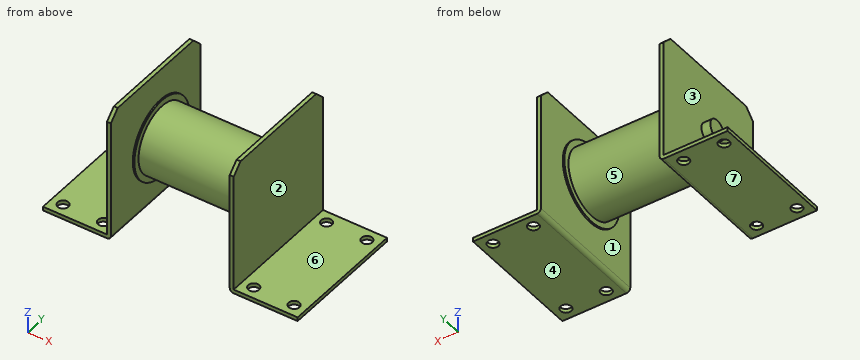
```python
from build123d import *

# Parameters (mm, degrees)
F0_R          = 20
F1_DEPTH      = 27.8
F1_DEPTH_BACK = 27.8
F2_R          = 7
F3_DEPTH      = 28.8
F3_DEPTH_BACK = 28.8
F4_R          = 20
F4_R_2        = 17
F5_DEPTH      = 27
F5_DEPTH_BACK = 27
F6_R          = 5
F7_DEPTH      = 32.2
F7_DEPTH_BACK = 36.7
F9_DEPTH      = 32.5
F9_DEPTH_BACK = 32.5
F10_SIZE      = 5
F11_R         = 2
F13_D         = 5.5


with BuildPart() as f1:
    # F0 (on Right) → F1 (new body, two sides)
    with BuildSketch(Plane.YZ) as f1_sk:
        Circle(F0_R)
    extrude(amount=F1_DEPTH)
    extrude(f1_sk.sketch, amount=-F1_DEPTH_BACK)

    # F2 (on Right) → F3 (join, two sides)
    with BuildSketch(Plane.YZ) as f3_sk:
        Circle(F2_R)
    extrude(amount=F3_DEPTH)
    extrude(f3_sk.sketch, amount=-F3_DEPTH_BACK)

    # F4 (on Right) → F5 (cut, two sides)
    with BuildSketch(Plane.YZ) as f5_sk:
        Circle(F4_R)
        Circle(F4_R_2, mode=Mode.SUBTRACT)
    extrude(amount=-F5_DEPTH, mode=Mode.SUBTRACT)
    extrude(f5_sk.sketch, amount=F5_DEPTH_BACK, mode=Mode.SUBTRACT)

    # F6 (on Right) → F7 (join, two sides)
    with BuildSketch(Plane.YZ) as f7_sk:
        Circle(F6_R)
    extrude(amount=F7_DEPTH)
    extrude(f7_sk.sketch, amount=-F7_DEPTH_BACK)

    # F8 (on Front) → F9 (join, two sides)
    with BuildSketch(Plane.XZ) as f9_sk:
        Polygon((32.2, 32.5), (30.2, 32.5), (30.2, -34.5), (64.7, -34.5), (64.7, -32.5), (32.2, -32.5), align=None)
        Polygon((-30.2, -34.5), (-30.2, 32.5), (-32.2, 32.5), (-32.2, -32.5), (-64.7, -32.5), (-64.7, -34.5), align=None)
    extrude(amount=F9_DEPTH)
    extrude(f9_sk.sketch, amount=-F9_DEPTH_BACK)

    # F10
    f10_edges = [f1.edges().sort_by_distance(p)[0] for p in [
        (31.2, -32.5, 32.5),
        (31.2, 32.5, 32.5),
        (-31.2, -32.5, 32.5),
        (-31.2, 32.5, 32.5),
    ]]
    chamfer(f10_edges, length=F10_SIZE)

    # F11
    f11_edges = [f1.edges().sort_by_distance(p)[0] for p in [
        (30.2, 0, -34.5),
        (-30.2, 0, -34.5),
    ]]
    fillet(f11_edges, radius=F11_R)

    # F13 (through all)
    with Locations(Plane.XY.offset(-32.5)):
        with Locations((38.2, 26.5), (38.2, -26.5), (58.7, -26.5), (-38.2, -26.5), (-58.7, -26.5), (-58.7, 26.5), (-38.2, 26.5), (58.7, 26.5)):
            Hole(F13_D / 2)


solid = f1.part
```
CAD build for the part. Positions are in the model's coordinates, mm. Face numbers are marked on the shaded views. A direction names the side the tool comes from. Round coordinates to 2 decimals unless told otherwise and drop trailing zeros. Write each loop counter-clockwise with the first axis right and the second up, starting at its lowest first coordinate (ties: lowest second). Pieces come first, ordered by that corner, then holes. Notation, with made-up numbers: (43.25, 28) - (100.25, 28) arc R23 ccw to (100.25, 45) - close; hole circle Ø1 at (35, 47.25). An arc over 180 degrees is marked (long way). Return JSON: item names as keys, results as strings. Group by question number.
Item 1: Probe probe 1 along X at (y, z) = (-3, 5.5); probe 2 along X at (y, z) = (3, 8); probe 3 along Y at (x, z) = (-38.2, -33.45). List the from-to ranges inside material, lowest first.
Item 2: Band-saw the part on B-B on z = 24. List the corners of the cut face in (x, y), plus the area to 3 significant figures.
Item 3: 3-axis set-ups, long thin cutter, end or side, ignore diameter. For the marked faces 5, 6 and 7: which of +Z, -Z, +X, -X, +Y, -Y reach the whole face in a straight line?
Item 4: Band-saw the part on A-A on x = 38.2. List the corners of the cut face in (y, z).
Item 5: Mould opens along X. For the marked faces 1, 2, 3 and 4 say: +X half, -X half, draft (parallel to the pull), parting line (faces both ways), or undercut.
Item 6: Flat gauge pins, fed straight in: pin 1 Ø5 at (y, z) = (-13.5, -14.5) entering from +X; pin 2 Ø10 at (x, z) = (-21.5, -3) entering from +Y; pin 3 Ø5 at (x, y) = (-38.2, 26.5) entering from +Z; pin 4 Ø6 at (x, y) = (0.5, 11) entering from -Z. Where does each tip first touch, or does it go through?
Item 7: Band-saw the part on C-C on y = -9.5. List the corners of the cut face in (x, z).
Item 8: Band-saw the part on D-D on x = -15.5. List the corners of the cut face in (y, z), plus the area to 3 significant figures.
Resolved:
{
 "1": {"probe 1": "x = -32.2 to -30.2, -28.8 to 28.8, 30.2 to 32.2", "probe 2": "x = -32.2 to -30.2, -27.8 to 27.8, 30.2 to 32.2", "probe 3": "y = -32.5 to -29.25, -23.75 to 23.75, 29.25 to 32.5"},
 "2": {"outline": "(-32.2, -32.5) - (-30.2, -32.5) - (-30.2, 32.5) - (-32.2, 32.5) - close; (30.2, -32.5) - (32.2, -32.5) - (32.2, 32.5) - (30.2, 32.5) - close", "area": "260 mm²"},
 "3": {"face 5": "none", "face 6": "+Z, +X, +Y, -Y", "face 7": "-Z, +X, -X, +Y, -Y"},
 "4": {"outline": "(-32.5, -34.5) - (-29.25, -34.5) - (-29.25, -32.5) - (-32.5, -32.5) - close; (-23.75, -34.5) - (23.75, -34.5) - (23.75, -32.5) - (-23.75, -32.5) - close; (29.25, -34.5) - (32.5, -34.5) - (32.5, -32.5) - (29.25, -32.5) - close"},
 "5": {"face 1": "undercut", "face 2": "+X half", "face 3": "-X half", "face 4": "draft"},
 "6": {"pin 1": "stops at x = 32.2", "pin 2": "stops at y = 17", "pin 3": "passes through", "pin 4": "stops at z = -15"},
 "7": {"outline": "(-64.7, -34.5) - (-32.2, -34.5) arc R2 ccw to (-30.2, -32.5) - (-30.2, 32.5) - (-32.2, 32.5) - (-32.2, -32.5) - (-64.7, -32.5) - close; (-27.8, -17.6) - (-27, -17.6) - (-27, -14.1) - (27, -14.1) - (27, -17.6) - (27.8, -17.6) - (27.8, 17.6) - (27, 17.6) - (27, 14.1) - (-27, 14.1) - (-27, 17.6) - (-27.8, 17.6) - close; (30.2, -32.5) arc R2 ccw to (32.2, -34.5) - (64.7, -34.5) - (64.7, -32.5) - (32.2, -32.5) - (32.2, 32.5) - (30.2, 32.5) - close"},
 "8": {"outline": "circle Ø34 at (0, 0)", "area": "908 mm²"}
}
